Autodesk Fusion 360 part; units mm, degrees
sketch "Sketch1" plane through (0, 0, 0) normal (0, 1, 0) x (1, 0, 0)
  line L0 (0, 0) -> (16.6, 0)
  line L1 (16.6, 0) -> (16.6, -16.6)
  line L2 (16.6, -16.6) -> (0, -16.6)
  line L3 (0, -16.6) -> (0, 0)
  line L4 (16.6, -16.6) -> (8.3, -16.6)
  line L5 (8.3, -16.6) -> (8.3, -11.7) construction
  circle A0 centre (8.3, -11.7) radius 4.5
  line L6 (16.6, -16.6) -> (15.3, -16.6)
  line L7 (16.6, -16.6) -> (16.6, -15.3)
  line L8 (15.3, -16.6) -> (15.3, -14) construction
  line L9 (16.6, -15.3) -> (14, -15.3) construction
  circle A1 centre (15.3, -15.3) radius 1
  circle A2 centre (1.3, -15.3) radius 1
  line L10 (0, -8.3) -> (16.6, -8.3) construction
  circle A3 centre (15.3, -1.3) radius 1
  circle A4 centre (1.3, -1.3) radius 1
  line L11 (8.3, 0) -> (8.3, -3.6)
  line L12 (5.5, -1) -> (11.1, -1)
  line L13 (11.1, -1) -> (11.1, -3.6)
  line L14 (11.1, -3.6) -> (5.5, -3.6)
  line L15 (5.5, -3.6) -> (5.5, -1)
  line L16 (13.6, 0) -> (13.6, -5.6) construction
  line L17 (16.6, -5.8) -> (13.6, -5.8) construction
  line L18 (14.6, -2.8) -> (12.6, -2.8)
  line L19 (12.6, -2.8) -> (12.6, -5.8)
  line L20 (12.6, -5.8) -> (14.6, -5.8)
  line L21 (14.6, -5.8) -> (14.6, -2.8)
  line L22 (3.0224, 0) -> (3.0224, -2.2) construction
  line L23 (0, -2.5501) -> (2.6, -2.5501) construction
  line L24 (2.6, -2.2) -> (4.9, -2.2)
  line L25 (4.9, -2.2) -> (4.9, -3.6)
  line L26 (4.9, -3.6) -> (2.6, -3.6)
  line L27 (2.6, -3.6) -> (2.6, -2.2)
  line L28 (0, -5.4812) -> (1.5, -5.4812) construction
  line L29 (2, 0) -> (2, -4) construction
  line L30 (1.5, -4) -> (3, -4)
  line L31 (3, -4) -> (3, -6.4)
  line L32 (3, -6.4) -> (1.5, -6.4)
  line L33 (1.5, -6.4) -> (1.5, -4)
  line L34 (3.1, -4) -> (4.6, -4)
  line L35 (4.6, -4) -> (4.6, -6.4)
  line L36 (4.6, -6.4) -> (3.1, -6.4)
  line L37 (3.1, -6.4) -> (3.1, -4)
  line L38 (0, -6) -> (3.1, -6) construction
  line L39 (12.35, -5.95) -> (14.85, -5.95)
  line L40 (14.85, -5.95) -> (14.85, -7.45)
  line L41 (14.85, -7.45) -> (12.35, -7.45)
  line L42 (12.35, -7.45) -> (12.35, -5.95)
  line L43 (13.6, -5.8) -> (13.6, -5.95)
  dimension "d1" = 16.6
  dimension "d2" = 16.6
  dimension "d3" = 8.3
  dimension "d4" = 4.9
  dimension "d5" = 9
  dimension "d6" = 1.3
  dimension "d7" = 1.3
  dimension "d8" = 2
  dimension "d9" = 3.6
  dimension "d10" = 5.6
  dimension "d11" = 2.6
  dimension "d12" = 5.6
  dimension "d13" = 3
  dimension "d14" = 2
  dimension "d15" = 3
  dimension "d16" = 2.8
  dimension "d17" = 2.2
  dimension "d18" = 2.6
  dimension "d19" = 2.3
  dimension "d20" = 1.4
  dimension "d21" = 1.5
  dimension "d22" = 4
  dimension "d23" = 1.5
  dimension "d24" = 2.4
  dimension "d25" = 1.5
  dimension "d26" = 2.4
  dimension "d27" = 3.1
  dimension "d28" = 2.5
  dimension "d29" = 1.5
  dimension "d30" = 0.15
extrude "Extrude1" add sketch "Sketch1" along normal blind 2 contours L11 L12 L13 L14 | L11 L12 L14 L15 | L0 L1 L2 L3 L4 L6 L7 | A0 | L18 L19 L20 L21 | L39 L40 L41 L42 | L24 L25 L26 L27 | L30 L31 L32 L33 | L34 L35 L36 L37 makes body 1
extrude "Extrude2" add sketch "Sketch1" along normal blind 2.1 contours A0 bodies 1
extrude "Extrude3" cut sketch "Sketch1" along normal blind 0.05 contours A0 bodies 1
extrude "Extrude4" add sketch "Sketch1" against normal blind 0.5 contours L18 L19 L20 L21 | L39 L40 L41 L42 | L24 L25 L26 L27 | L30 L31 L32 L33 | L34 L35 L36 L37 bodies 1
extrude "Extrude5" add sketch "Sketch1" against normal blind 3 contours L11 L12 L13 L14 | L11 L12 L14 L15 bodies 1
sketch "Sketch2" plane through (0, -3, 0) normal (0, -1, 0) x (1, 0, 0)
  line L0 (11.1, 3.6) -> (5.5, 3.6)
  line L1 (5.5, 3.6) -> (5.5, 1)
  line L2 (5.5, 1) -> (11.1, 1)
  line L3 (11.1, 1) -> (11.1, 3.6)
  line L4 (5.5, 2.3) -> (11.1, 2.3)
  circle A0 centre (8.3, 2.3) radius 0.25
  line L5 (5.5, 2.3) -> (6.5, 2.3)
  circle A1 centre (6.5, 2.3) radius 0.25
  line L6 (11.1, 2.3) -> (10.1, 2.3)
  circle A2 centre (10.1, 2.3) radius 0.25
  circle A3 centre (6.5, 2.3) radius 0.75
  circle A4 centre (10.1, 2.3) radius 0.75
  line L7 (10.1, 3.05) -> (6.5, 3.05)
  line L8 (10.1, 1.55) -> (6.5, 1.55)
  dimension "d41" = 0.5
  dimension "d42" = 1
  dimension "d43" = 0.5
  dimension "d44" = 1
  dimension "d45" = 0.5
  dimension "d46" = 1.5
  dimension "d47" = 1.5
extrude "Extrude6" add sketch "Sketch2" along normal blind 3 separate body contours L4 L6 A2 A4 | L4 L6 A2 A4 | L4 L5 A1 A3 | L4 L5 A1 A3 | L4 A0 A3 A4 L7 | L4 A0 A3 A4 L8 makes body 2
extrude "Extrude7" add sketch "Sketch2" along normal blind 4.5 separate body contours L4 A0 A3 A4 L7 makes body 3
sketch "Sketch3" plane through (0, 0, 2.3) normal (0, 0, -1) x (-1, 0, 0)
  line L0 (-7.25, -3) -> (-8.05, -3)
  line L1 (-8.05, -3) -> (-8.05, -7.5)
  line L2 (-8.05, -7.5) -> (-7.25, -7.5)
  line L3 (-7.25, -7.5) -> (-7.25, -3)
  line L4 (-7.65, -7.5) -> (-8.3, -7.5)
  line L5 (-7.65, -7.5) -> (-6.5, -7.5)
  line L6 (-6.5, -7.5) -> (-6.5, -6.75)
  circle A0 centre (-6.5, -6.75) radius 0.75
  line L7 (-5.75, -6.75) -> (-5.75, -5.6822)
  line L8 (-5.75, -5.6822) -> (-6.7545, -6.0445)
  line L9 (-8.3, -7.5) -> (-10.1, -7.5)
  line L10 (-10.1, -7.5) -> (-10.1, -6.75)
  circle A1 centre (-10.1, -6.75) radius 0.75
  line L11 (-10.85, -6.75) -> (-10.85, -5.6967)
  line L12 (-10.85, -5.6967) -> (-9.8547, -6.0413)
  line L13 (-10.85, -5.6967) -> (-5.75, -5.6822)
  dimension "d52" = 0.65
  dimension "d53" = 1.15
  dimension "d54" = 0.75
  dimension "d55" = 1.5
  dimension "d56" = 1.8
  dimension "d57" = 0.75
  dimension "d58" = 1.5
delete_body "RemoveBody1" bodies 3
extrude "Extrude8" add sketch "Sketch3" along normal blind -0.75 and the other way blind -4 separate body contours L3 A0 L8 L13 | L1 L2 L3 L4 L5 L13 | L1 L4 L9 A1 L12 L13 | L3 L5 A0 | A0 | A0 L7 L8 | A1 L11 L12 | A1 makes body 4
extrude "Extrude9" cut 1 faces at (8.3062, -6, 1.7169) along direction (0, 1, 0) blind 1.75 on bodies 2 bodies 2
extrude "Extrude10" cut sketch "Sketch2" against normal blind 0.5 contours L0 L1 L3 L4 L5 L6 A3 A4 L7 | L1 L2 L3 L4 L5 L6 A3 A4 L8 bodies 1
move_body "Move1" bodies 4 to x (1, 0, 0) y (0, 1, 0) z (0, 0, 1) at (0, 1.75, 0)
combine "Combine1" operation add target body 1 tool bodies 2 4
CAD build for the part. Positions are in the model's coordinates, mm. A direction names the side the tool comes from. Coordinates: 2 decimals unless noted, no trailing zeros. Order: outer loops, then holes, each group sorted by start corner. A loop starts at its lowest first (then second) coordinate and runs counter-clockwise, first axis right, second up. Notation, with made-up numbers: (75, 62) - (112, 62) arc R10 cw to (112, 79) - close; hole circle Ø10 at (67.25, 68). An arc over 180 degrees is marked (long way). Use a Markdown table: item, result. Add a question column.
(1) Saw through at B-B (z = 1.3). Give the cut face in (x, y), then the cut area to 3 significant figures.
(2) Saw through at D-D (z = 11.7). Give the cut face in (x, y), then the cut area to 4 significant figures.
(3) Saw through at C-C (y = 1.25). Give the cut face in (x, z).
(4) Drill centre lines: line 1 along X through (y, z) = (-3.7, 2.3); line 2 along Z through (x, y) = (15.3, 1.35). Where is each one in solid material? Low to high. Write a range as [from, to].
(5) Pull direction Y, two halves, no side cores. Call faces 6 (the face through (5.75, -3.23, 2.32)), 7 (the face through (14, -0.5, 7)), 8 (the face through (5.5, -1, 2)), 9 (the face through (8.3, -2.5, 3.2)): +Y half, -Y half, draft (parallel to the pull), parting line (faces both ways), or undercut.
(6) Flat gauge pins, fed straight in: pin 1 (1 mm diameter, centred on y = -1.5, z = 1.5, fed in from +X); pin 2 (0.6 mm diameter, centred on y = -0.5, z = 5.5, fed in from +X); pin 3 (1.6 mm diameter, centred on x = 2, z = 5.5, fed in from -Y). Where does each tip first touch, or does it go through?
(7) Saw through at A-A (z = 15.3). Give the cut face in (x, y).
(8) Which spindle directions (+Z, -Z, +X, -X, +Y, -Y) get a long thin tool onto all of the face, cutting with end or side? Do faces 1 (the face through (4, -0.5, 3)), 2 (the face through (8, 1, 16.6)), 3 (the face through (16.254, 0.986, 1.6)), 4 (the face through (8, -1, 1)), 5 (the face through (10.85, -4.5, 0.6)). Say none if no direction does.
Solved:
| question | item | result |
|---|---|---|
| 1 | outline | (0, 0) - (0.3, 0) - (0.3, 2) - (0, 2) - close; (2.3, 0) - (5.5, 0) - (5.5, -2.5) - (11.1, -2.5) - (11.1, 0) - (14.3, 0) - (14.3, 2) - (2.3, 2) - close; (5.75, -5) arc R0.75 ccw to (6.5, -5.75) - (10.1, -5.75) arc R0.75 ccw to (10.85, -5) - (10.85, -3.95) - (5.75, -3.93) - close; (16.3, 0) - (16.6, 0) - (16.6, 2) - (16.3, 2) - close |
| 1 | area | 48.2 mm² |
| 2 | outline | (0, 0) - (3.8, 0) - (3.8, 0.05) - (12.8, 0.05) - (12.8, 0) - (16.6, 0) - (16.6, 2) - (12.8, 2) - (12.8, 2.1) - (3.8, 2.1) - (3.8, 2) - (0, 2) - close |
| 2 | area | 33.65 mm² |
| 3 | outline | (0, 0) - (16.6, 0) - (16.6, 16.6) - (0, 16.6) - close; hole circle Ø2 at (1.3, 1.3); hole circle Ø2 at (1.3, 15.3); hole circle Ø2 at (15.3, 1.3); hole circle Ø2 at (15.3, 15.3) |
| 4 | line 1 | x = [5.75, 6.25], [6.75, 8.05], [8.55, 9.85], [10.35, 10.85] |
| 4 | line 2 | z = [0, 0.3], [2.3, 14.3], [16.3, 16.6] |
| 5 | face 6 | undercut |
| 5 | face 7 | -Y half |
| 5 | face 8 | draft |
| 5 | face 9 | undercut |
| 6 | pin 1 | stops at x = 11.1 |
| 6 | pin 2 | stops at x = 14.6 |
| 6 | pin 3 | stops at y = -0.5 |
| 7 | outline | (0, 0) - (0.3, 0) - (0.3, 2) - (0, 2) - close; (2.3, 0) - (5.6, 0) - (5.6, 0.05) - (11, 0.05) - (11, 0) - (14.3, 0) - (14.3, 2) - (11, 2) - (11, 2.1) - (5.6, 2.1) - (5.6, 2) - (2.3, 2) - close; (16.3, 0) - (16.6, 0) - (16.6, 2) - (16.3, 2) - close |
| 8 | face 1 | +Z, -Z, -X, -Y |
| 8 | face 2 | +Z, +X, -X, +Y, -Y |
| 8 | face 3 | +Y, -Y |
| 8 | face 4 | -Z, +X, -X |
| 8 | face 5 | +Z, -Z, +X, -Y |
